The figure shows three views and two pictorial views of one solid part (mm, origin at its lowest corner). Answer the questions. A direction names the side the tool comes from. Round coordinates to 2 decimals unless told otherwise and drop trailing zeros. Order: outer loops, then holes, each group sorted by start corner. A loop starts at its lowest first (then second) coordinate and runs counter-clockwise, first axis right, second up. Notation, with made-up numbers: (31.25, -12.5) - (52.25, -12.5) arc R27 ccw to (52.25, 17.5) - close; hole circle Ø1 at (86.25, -23.5). An arc over 180 degrees is marked (long way). Answer in a Markdown table with one row per item.
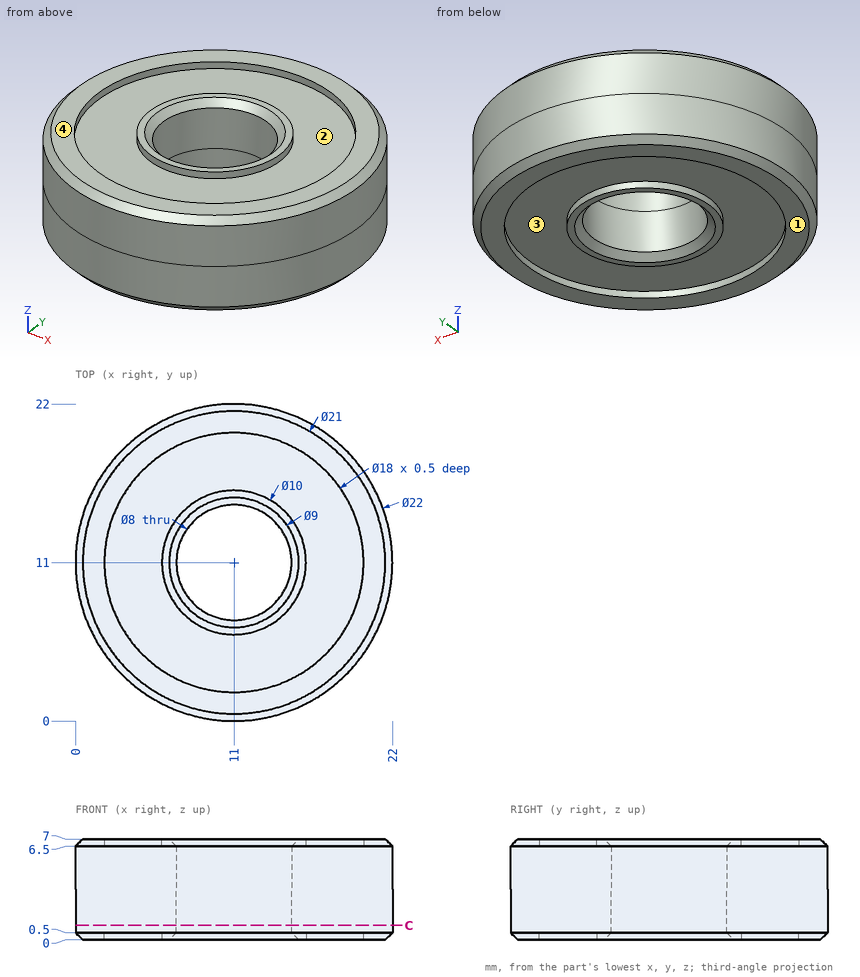
1) The mould has two halves that part along Y. Classify the marked faces 1 and 2: released by +Y, released by -Y, zero draft, split by the parting line, or undercut.
Filled in:
| item | result |
|---|---|
| face 1 | zero draft |
| face 2 | undercut |
2) Find section C-C, the plane z = 1. Give the vertices of the cut face in (x, y).
Filled in:
| item | result |
|---|---|
| outline | circle Ø22 at (11, 11); hole circle Ø8 at (11, 11) |
3) Each of these flat-tipped pins is pushed along its axis until it touches: pin 1 (7 mm diameter, centred on x = 11, y = 11, fed in from -Z); pin 2 (4 mm diameter, centred on x = 15, z = 5, fed in from -Y); pin 3 (2 mm diameter, centred on x = 4.5, z = 6, fed in from -Y). Where does it stop, or does it pass through?
Filled in:
| item | result |
|---|---|
| pin 1 | passes through |
| pin 2 | stops at y = 0.18 |
| pin 3 | stops at y = 1.47 |
4) Which of the six approach directions +Z, -Z, +X, -X, +Y, -Y give full straight-line access (tool end or side, diameter ignored) to the marked faces 3 and 4?
Filled in:
| item | result |
|---|---|
| face 3 | -Z |
| face 4 | +Z, +X, -X, +Y, -Y |
5) Find the intervals of material crossed by probe 1 along Y at (x, z) = (11, 1.85); probe 2 along Y at (x, z) = (11, 0.2); probe 3 along Z at (x, y) = (5.5, 14), in increasing order. Write a range as from..to.
Filled in:
| item | result |
|---|---|
| probe 1 | y = 0..7, 15..22 |
| probe 2 | y = 0.3..2, 6..6.7, 15.3..16, 20..21.7 |
| probe 3 | z = 0.5..6.5 |
